Input: part model. Units: mm. Frame: model coordinates. Face numbers are marked on the shaded views. A direction names the side the tool comes from. Round coordinates to 2 decimals unless told otherwise and drop trailing zeros. Order: outer loops, then holes, each group sorted by start corner. A loop starts at its lowest first (then second) coordinate and runs counter-clockwise, first axis right, second up. Notation, with made-up numbers: (63, -10.5) -> (74, -10.5) arc R27 cw to (74, 19.5) -> close; hole circle Ø6 at (53.25, 41.25). An arc over 180 degrees is marked (long way). Use a Markdown table: item, result.
from build123d import *

# Parameters (mm, degrees)
F0_W     = 57.15
F0_H     = 44.45
F1_DEPTH = 25.4
F3_DEPTH = 25.401
F5_DEPTH = 12.7


with BuildPart() as f1:
    # F0 (on Front) → F1 (new body)
    with BuildSketch(Plane.XZ):
        with Locations((-1.039090705, 22.225)):
            Rectangle(F0_W, F0_H)
    extrude(amount=F1_DEPTH)

    # F2 (on face) → F3 (cut, through all)
    with BuildSketch(Plane.XZ.offset(25.4)):
        with BuildLine():
            Line((-4.214090705, 33.3375), (-4.214090705, 34.925))
            ThreePointArc((-4.214090705, 34.925), (-4.6590277858, 34.9172035516), (-5.1034185785, 34.8938237786))
            Line((-5.1034185785, 34.8938237786), (-4.214090705, 33.3375))
        make_face()
        with BuildLine():
            Line((6.2490833223, 15.0269454522), (-4.214090705, 33.3375))
            Line((-4.214090705, 33.3375), (-4.214090705, 9.525))
            ThreePointArc((-4.214090705, 9.525), (1.6966921214, 10.984330697), (6.2490833223, 15.0269454522))
        make_face()
        with BuildLine():
            ThreePointArc((8.485909295, 22.225), (4.7661654161, 31.2052561211), (-4.214090705, 34.925))
            Line((-4.214090705, 34.925), (-4.214090705, 33.3375))
            Line((-4.214090705, 33.3375), (6.2490833223, 15.0269454522))
            ThreePointArc((6.2490833223, 15.0269454522), (7.9138174029, 18.4562011295), (8.485909295, 22.225))
        make_face()
        with BuildLine():
            Line((-4.214090705, 9.525), (-4.214090705, 33.3375))
            Line((-4.214090705, 33.3375), (-5.1034185785, 34.8938237786))
            ThreePointArc((-5.1034185785, 34.8938237786), (-16.9062942566, 21.7800629192), (-4.214090705, 9.525))
        make_face()
    extrude(amount=-F3_DEPTH, mode=Mode.SUBTRACT)

    # F4 (on face) → F5 (cut)
    with BuildSketch(Plane.XZ.offset(25.4)):
        with BuildLine():
            Line((6.2490833223, 15.0269454522), (14.835909295, 0))
            Line((14.835909295, 0), (27.535909295, 0))
            Line((27.535909295, 0), (27.535909295, 44.45))
            Line((27.535909295, 44.45), (-10.564090705, 44.45))
            Line((-10.564090705, 44.45), (-5.1034185785, 34.8938237786))
            ThreePointArc((-5.1034185785, 34.8938237786), (4.4460344675, 31.5143612265), (8.485909295, 22.225))
            ThreePointArc((8.485909295, 22.225), (7.9138174029, 18.4562011295), (6.2490833223, 15.0269454522))
        make_face()
    extrude(amount=-F5_DEPTH, mode=Mode.SUBTRACT)


solid = f1.part
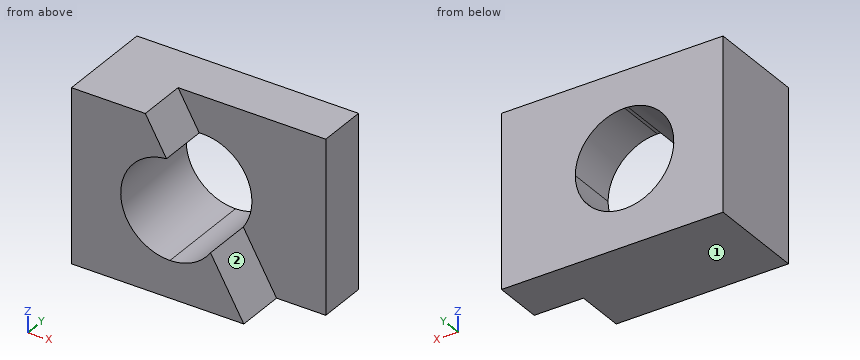
1) Set-up query: the marked faces 1 and 2. Return all of +Z, -Z, +X, -X, +Y, -Y with unobstructed straight access to the full face (end or side cutting, diameter ignored); none if empty.
Answer key:
| item | result |
|---|---|
| face 1 | -Z, +X, -X, +Y, -Y |
| face 2 | +Z, +X, -Y |
2) Cut plane A-A on y = -3.25. Return loops of the section in (x, z) (3 decimals).
Answer key:
| item | result |
|---|---|
| outline | (-29.614, 0) -> (27.536, 0) -> (27.536, 44.45) -> (-29.614, 44.45) -> close; hole circle Ø25.4 at (-4.214, 22.225) |
3) Cut plane B-B on z = 16. Return loops of the section in (x, y).
Answer key:
| item | result |
|---|---|
| outline | (-29.61, -25.4) -> (-15.28, -25.4) -> (-15.28, 0) -> (-29.61, 0) -> close; (6.86, -12.7) -> (27.54, -12.7) -> (27.54, 0) -> (6.86, 0) -> close |
4) Ray query, probe 1 along Y at (x, z) = (15.5, 23); probe 2 along Z at (x, y) = (-13.5, -2.25); probe 3 along Z at (x, y) = (-15, -10.25). Return the intervals inside material, ascending.
Answer key:
| item | result |
|---|---|
| probe 1 | y = -12.7 to 0 |
| probe 2 | z = 0 to 13.56, 30.89 to 44.45 |
| probe 3 | z = 0 to 15.52, 28.93 to 44.45 |
5) Cut plane D-D on y = -19.75. Return loops of the section in (x, z) (3 decimals), and give its area (3 significant figures).
Answer key:
| item | result |
|---|---|
| outline | (-29.614, 0) -> (14.836, 0) -> (6.249, 15.027) arc R12.7 cw (long way) to (-5.103, 34.894) -> (-10.564, 44.45) -> (-29.614, 44.45) -> close |
| area | 1,020 mm^2 |
6) Cut plane C-C on x = -6.5. Return loops of the section in (y, z).
Answer key:
| item | result |
|---|---|
| outline | (-25.4, 0) -> (0, 0) -> (0, 9.73) -> (-25.4, 9.73) -> close; (-25.4, 34.72) -> (0, 34.72) -> (0, 44.45) -> (-12.7, 44.45) -> (-12.7, 37.34) -> (-25.4, 37.34) -> close |
